Here's how the part is built. I have some questions about the finished solid (model axes, mm). Face numbers are marked on the shaded views. A direction names the side the tool comes from. Coordinates: 2 decimals unless noted, no trailing zeros. Write each loop counter-clockwise with the first axis right and the second up, starting at its lowest first coordinate (ties: lowest second). Pieces come first, ordered by that corner, then holes. Notation, with made-up numbers: (73, 75) -> (84, 75) arc R5 cw to (84, 84) -> close; hole circle Ø1 at (-18.5, 15). An arc over 180 degrees is marked (long way). Answer in a Markdown table with one row per item. Add a question column.
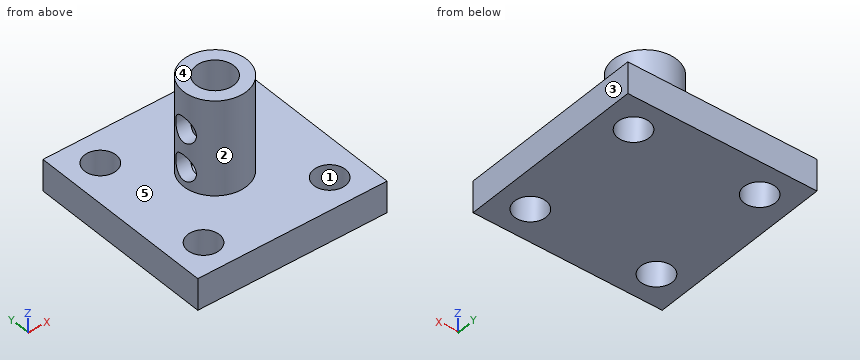
from build123d import *

# Parameters (mm, degrees)
ESBO_O1_W                = 30
ESBO_O1_H                = 30
ESBO_O1_R                = 2.5
RESSALTO_EXTRUS_O1_DEPTH = 5
ESBO_O3_R                = 5
RESSALTO_EXTRUS_O2_DEPTH = 15
ESBO_O4_R                = 3
CORTE_EXTRUS_O1_DEPTH    = 15
ESBO_O5_R                = 2
CORTE_EXTRUS_O2_DEPTH    = 15


with BuildPart() as part:
    # Esboço1 → Ressalto-extrusão1 (new body)
    with BuildSketch(Plane.XY):
        Rectangle(ESBO_O1_W, ESBO_O1_H)
        with Locations((-10, 10)):
            Circle(ESBO_O1_R, mode=Mode.SUBTRACT)
        with Locations((10, 10)):
            Circle(ESBO_O1_R, mode=Mode.SUBTRACT)
        with Locations((10, -10)):
            Circle(ESBO_O1_R, mode=Mode.SUBTRACT)
        with Locations((-10, -10)):
            Circle(ESBO_O1_R, mode=Mode.SUBTRACT)
    extrude(amount=RESSALTO_EXTRUS_O1_DEPTH)

    # Esboço3 → Ressalto-extrusão2 (add)
    with BuildSketch(Plane.XY.offset(5)):
        Circle(ESBO_O3_R)
    extrude(amount=RESSALTO_EXTRUS_O2_DEPTH)

    # Esboço4 → Corte-extrusão1 (cut)
    with BuildSketch(Plane.XY.offset(20)):
        Circle(ESBO_O4_R)
    extrude(amount=-CORTE_EXTRUS_O1_DEPTH, mode=Mode.SUBTRACT)

    # Esboço5 → Corte-extrusão2 (cut)
    with BuildSketch(Plane(origin=(0, 0, 0), x_dir=(0, 0, -1), z_dir=(1, 0, 0))):
        with Locations((-8, 0)):
            Circle(ESBO_O5_R)
        with Locations((-14, 0)):
            Circle(ESBO_O5_R)
    extrude(amount=-CORTE_EXTRUS_O2_DEPTH, mode=Mode.SUBTRACT)


solid = part.part
Q1. Imagine slicing it at D-D on z = 11.25. Please give me the cut outline in (x, y).
Q2. For the marked faces 4 and 5, which set-ups out of +Z, -Z, +X, -X, +Y, -Y let a thin tool reach every point of the face, with its end or its side?
Q3. Imagine slicing it at C-C on x = -4.25. Please give me the cut outline in (y, z).
Q4. Imagine slicing it at A-A on x = -10. Please give me the cut outline in (y, z).
Q5. I need wall thicknesses on line 1 (Y direction, x = -10, z = 3.1); line 2 (Y direction, x = 0, z = 16.75); line 3 (Y direction, x = -11.5, z = 1). Which ranges of each line are inside material? Lowest first, please. Write a range as [from, to].
Q6. I'm going to push flat-ended pins straight in: P1, Ø4.5, axis at y = 0, z = 8, coming from the +X side; P2, Ø6.5, axis at y = 0, z = 14, coming from the -X side; P3, Ø1.8, axis at x = 1, y = -1.5, coming from the +Z side; P4, Ø4, axis at x = 10, y = -10, coming from the -Z side. Where does each tip first touch, or does it pass through?
Q7. If we mould it in two halves opening along X, with no side actions, what happens to the marked faces 1, 2 and 3? For each: pulls with the +X half, pulls with the -X half, needs draft (parallel to the pull), parting line crosses it, or undercut.
Result sheet:
| question | item | result |
|---|---|---|
| 1 | outline | circle Ø10 at (0, 0); hole circle Ø6 at (0, 0) |
| 2 | face 4 | +Z, +X, -X, +Y, -Y |
| 2 | face 5 | +Z |
| 3 | outline | (-15, 0) -> (15, 0) -> (15, 5) -> (2.63, 5) -> (2.63, 20) -> (-2.63, 20) -> (-2.63, 5) -> (-15, 5) -> close; hole circle Ø4 at (0, 8); hole circle Ø4 at (0, 14) |
| 4 | outline | (-15, 0) -> (-12.5, 0) -> (-12.5, 5) -> (-15, 5) -> close; (-7.5, 0) -> (7.5, 0) -> (7.5, 5) -> (-7.5, 5) -> close; (12.5, 0) -> (15, 0) -> (15, 5) -> (12.5, 5) -> close |
| 5 | line 1 | y = [-15, -12.5], [-7.5, 7.5], [12.5, 15] |
| 5 | line 2 | y = [-5, -3], [3, 5] |
| 5 | line 3 | y = [-15, -12], [-8, 8], [12, 15] |
| 6 | P1 | stops at x = 5 |
| 6 | P2 | stops at x = -5 |
| 6 | P3 | stops at z = 5 |
| 6 | P4 | passes through |
| 7 | face 1 | undercut |
| 7 | face 2 | parting line crosses it |
| 7 | face 3 | pulls with the +X half |
